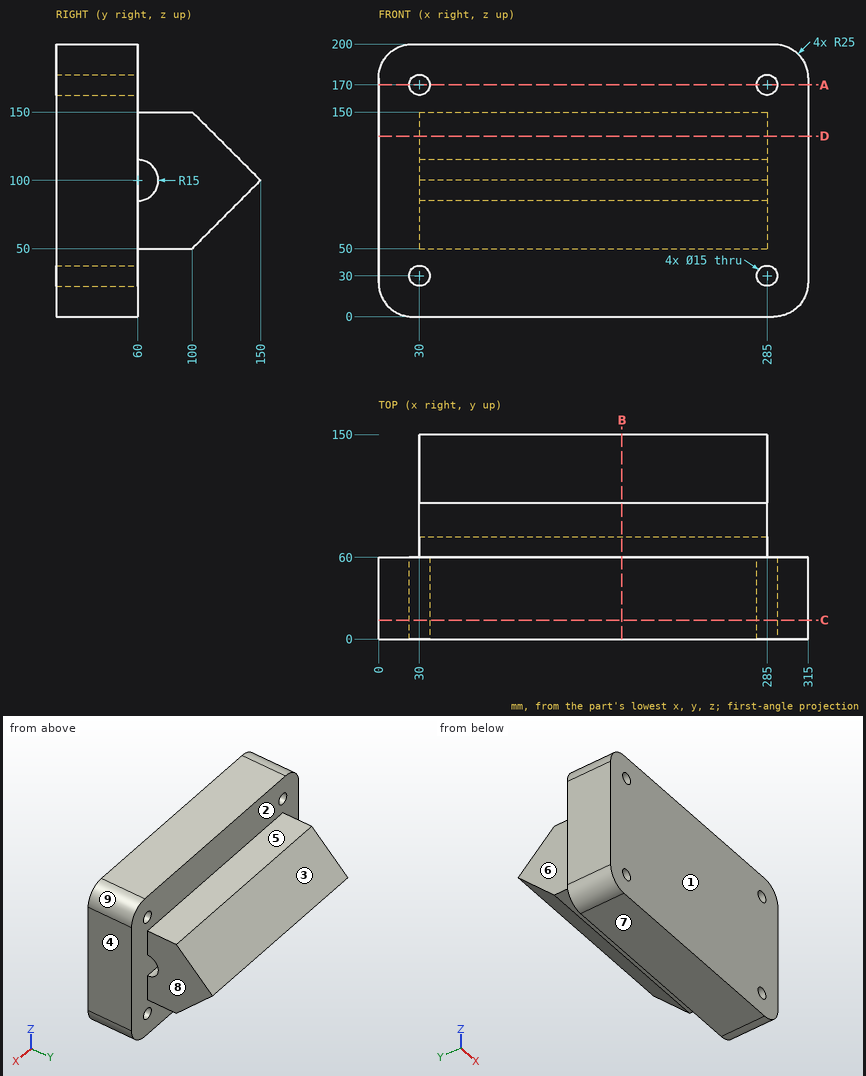
Print and shaded views of the part. All mm, measured from the part's lowest x, y and z. A direction names the side the tool comes from. Give positions to 0.01 mm unless a question says otherwise; leave off trailing zeros. Loops run counter-clockwise (first coordinate to the right, second up) from the corner with the lowest first, then second, coordinate; pieces in that order, holes last. Notation, with made-up numbers: (14, 44.25) - (23, 44.25) arc R23 cw to (23, 58.25) - close; hole circle Ø6 at (76.5, 37.25). An arc over 180 degrees is marked (long way). Use a Markdown table: item, result.
(1) Wall check: line 1 along X through (y, z) = (21, 30); line 2 along Z through (x, y) = (30, 19.5); line 3 along X through (y, z) = (26.5, 173). Give the ranges that are in metal, low to high.
Taken from the geometry:
| item | result |
|---|---|
| line 1 | 0 to 22.5, 37.5 to 277.5, 292.5 to 315 |
| line 2 | 0 to 22.5, 37.5 to 162.5, 177.5 to 200 |
| line 3 | 0 to 23.13, 36.87 to 278.13, 291.87 to 315 |
(2) Drop flat-ended pins along their axis: pin 1 Ø5 at (x, z) = (220.5, 39) entering from +Y; pin 2 Ø3 at (x, z) = (259.5, 118.5) entering from +Y; pin 3 Ø2 at (y, z) = (68, 128) entering from +X. Give the stop position or say it passes through.
Taken from the geometry:
| item | result |
|---|---|
| pin 1 | y = 60 |
| pin 2 | y = 133 |
| pin 3 | x = 285 |
(3) Band-saw the part on A-A (z = 170). Give the cut face in (x, y), and give its area (3 significant figures).
Taken from the geometry:
| item | result |
|---|---|
| outline | (0, 0) - (22.5, 0) - (22.5, 60) - (0, 60) - close; (37.5, 0) - (277.5, 0) - (277.5, 60) - (37.5, 60) - close; (292.5, 0) - (315, 0) - (315, 60) - (292.5, 60) - close |
| area | 17,100 mm2 |
(4) Band-saw the part on C-C (y = 14). Give the cut face in (x, z), and give its area (3 significant figures).
Taken from the geometry:
| item | result |
|---|---|
| outline | (0, 25) arc R25 ccw to (25, 0) - (290, 0) arc R25 ccw to (315, 25) - (315, 175) arc R25 ccw to (290, 200) - (25, 200) arc R25 ccw to (0, 175) - close; hole circle Ø15 at (30, 30); hole circle Ø15 at (30, 170); hole circle Ø15 at (285, 30); hole circle Ø15 at (285, 170) |
| area | 61,800 mm2 |
(5) Pull direction Y, two halves, no side cores. Call the marked faces 1, 2, 3 and 4: +Y half, -Y half, draft (parallel to the pull), parting line (faces both ways), or undercut.
Taken from the geometry:
| item | result |
|---|---|
| face 1 | -Y half |
| face 2 | undercut |
| face 3 | +Y half |
| face 4 | draft |
(6) Band-saw the part on D-D (z = 132.5). Give the cut face in (x, y), and give its area (3 significant figures).
Taken from the geometry:
| item | result |
|---|---|
| outline | (0, 0) - (315, 0) - (315, 60) - (285, 60) - (285, 117.5) - (30, 117.5) - (30, 60) - (0, 60) - close |
| area | 33,600 mm2 |
(7) Band-saw the part on B-B (x = 178.5). Give the cut face in (y, z).
Taken from the geometry:
| item | result |
|---|---|
| outline | (0, 0) - (60, 0) - (60, 50) - (100, 50) - (150, 100) - (100, 150) - (60, 150) - (60, 200) - (0, 200) - close; hole (60, 85) arc R15 ccw to (60, 115) - close |
(8) Which spindle directions (+Z, -Z, +X, -X, +Y, -Y) get a long thin tool onto all of the face, cutting with end or side? Do the marked faces 5, 6, 7, 8 and 9. Say none if no direction does.
Taken from the geometry:
| item | result |
|---|---|
| face 5 | +Z, +X, -X, +Y |
| face 6 | +Z, -Z, -X, +Y |
| face 7 | -Z, +X, -X, +Y, -Y |
| face 8 | +Z, -Z, +X, +Y |
| face 9 | +Z, +X, +Y, -Y |
